Geometry: final body of the model. Coordinates: model frame, mm. A direction names the side the tool comes from. Coordinates: 2 decimals unless noted, no trailing zeros. Write each loop counter-clockwise with the first axis right and the second up, starting at its lowest first coordinate (ties: lowest second). Pieces come first, ordered by that corner, then holes. Notation, with made-up numbers: (2, 75.25) - (24, 75.25) arc R13 cw to (24, 86.25) - close; hole circle Ø6 at (-18, 33.5). An arc over 180 degrees is marked (long way). Answer as a JSON object with one key per item and string values. Group by question number.
Item 1: Section D-D on x = 16.25. Return loops of the section in (y, z).
Item 2: Set-up query: faces 1 (the flat face through (20.419, -10.108, 0.986)), 2 (the flat face through (7, 1, 0)), 3 (the flat face through (11, -14.5, 8)), 4 (the flat face through (17.875, 0, 8)), 5 (the flat face through (16, -1.5, 8)). Return all of +Z, -Z, +X, -X, +Y, -Y with unobstructed straight access to the full face (end or side cutting, diameter ignored); none if empty.
Item 3: Section A-A on z = 3.25. Return loops of the section in (x, y) (3 decimals).
Item 4: Mould query, pull axis X, two halves, no side actions, for faces 6 (the flat face through (11, 13, 8)), 7 (the flat face through (14.875, 0, 8)), 8 (the cylindrical face through (2.8, -45.89, 0.99)), 9 (the cylindrical face through (8.19, 48.22, 1.01)). Classes: pulls with the +X half, pulls with the -X half, needs draft (parallel to the pull), parting line crosses it, or undercut.
Item 5: Line query: line 1 along Y through (x, z) = (3, 1.6); line 2 along Y through (x, z) = (11, 3.5); line 3 along Z through (x, y) = (2.5, 29.5). Output: solid intervals per line, ascending. Write a range as from..to.
Item 6: Section B-B on y = 0. Return loops of the section in (x, z) (3 decimals), and give its area (3 significant figures).
Item 7: Section C-C on x = 3. Return loops of the section in (y, z), and give its area (3 significant figures).
Item 8: First-contact query: pin 1 Ø2 at (x, z) = (18.5, 13) entering from +Y; pin 2 Ø0.9 at (x, z) = (16.5, 11.5) entering from +Y; pin 3 Ø6 at (x, z) = (12, 9.5) entering from -Y. Flat tips, straight axial feed; report the tip coordinate or a pass-through.
```python
from build123d import *

# Parameters (mm, degrees)
SKETCH1_R           = 1.5
BOSS_EXTRUDE1_DEPTH = 2
FILLET1_R           = 15
FILLET2_R           = 3
FILLET3_R           = 1.5
FILLET4_R           = 5
SKETCH2_W           = 1.5
SKETCH2_H           = 3
SKETCH2_W_2         = 0.75
BOSS_EXTRUDE2_DEPTH = 13
SKETCH4_W           = 3
SKETCH4_H           = 29
CUT_EXTRUDE1_DEPTH  = 13


with BuildPart() as part:
    # Sketch1 → Boss-Extrude1 (new body)
    with BuildSketch(Plane.XY):
        Polygon((0, 52.37615434), (0, -52.37615434), (8.5, -48.47615434), (13, -20), (28, 0), (13, 20), (8.5, 48.47615434), align=None)
        with Locations((3, -47.37615434)):
            Circle(SKETCH1_R, mode=Mode.SUBTRACT)
        with Locations((22.62384566, 0)):
            Circle(SKETCH1_R, mode=Mode.SUBTRACT)
        with Locations(Location((3, 47.37615434, 0), (0, 0, 180))):
            Circle(SKETCH1_R, mode=Mode.SUBTRACT)
    extrude(amount=BOSS_EXTRUDE1_DEPTH)

    # Fillet1
    fillet1_edges = [part.edges().sort_by_distance(p)[0] for p in [
        (13, 20, 1),
        (13, -20, 1),
    ]]
    fillet(fillet1_edges, radius=FILLET1_R)

    # Fillet2
    fillet2_edges = [part.edges().sort_by_distance(p)[0] for p in [
        (8.5, 48.47615434, 1),
        (8.5, -48.47615434, 1),
    ]]
    fillet(fillet2_edges, radius=FILLET2_R)

    # Fillet3
    fillet3_edges = [part.edges().sort_by_distance(p)[0] for p in [
        (0, -52.37615434, 1),
        (0, 52.37615434, 1),
    ]]
    fillet(fillet3_edges, radius=FILLET3_R)

    # Fillet4
    fillet4_edges = [part.edges().sort_by_distance(p)[0] for p in [
        (28, 0, 1),
    ]]
    fillet(fillet4_edges, radius=FILLET4_R)

    # Sketch2 → Boss-Extrude2 (add)
    with BuildSketch(Plane.XY.offset(2)):
        Polygon((17.125, 13), (17.125, 14.5), (0, 14.5), (0, -14.5), (17.125, -14.5), (17.125, -13), (15.625, -13), (1.5, -13), (1.5, 13), (15.625, 13), align=None)
        with Locations((16.375, 0)):
            Rectangle(SKETCH2_W, SKETCH2_H)
        with Locations((17.5, 0)):
            Rectangle(SKETCH2_W_2, SKETCH2_H)
        with Locations((15.25, 0)):
            Rectangle(SKETCH2_W_2, SKETCH2_H)
    extrude(amount=BOSS_EXTRUDE2_DEPTH)

    # Sketch4 → Cut-Extrude1 (cut)
    with BuildSketch(Plane.XY.offset(15)):
        with Locations((3, 0)):
            Rectangle(SKETCH4_W, SKETCH4_H)
    extrude(amount=-CUT_EXTRUDE1_DEPTH, mode=Mode.SUBTRACT)


solid = part.part
```
Checks:
{
 "1": {"outline": "(-15.67, 0) - (15.67, 0) - (15.67, 2) - (14.5, 2) - (14.5, 15) - (13, 15) - (13, 2) - (1.5, 2) - (1.5, 15) - (-1.5, 15) - (-1.5, 2) - (-13, 2) - (-13, 15) - (-14.5, 15) - (-14.5, 2) - (-15.67, 2) - close"},
 "2": {"face 1": "+Z, -Z, +X, -Y", "face 2": "-Z, +X, -X, +Y, -Y", "face 3": "+Z, +X, -X, -Y", "face 4": "+Z, +X, +Y, -Y", "face 5": "+Z, +X"},
 "3": {"outline": "(0, -14.5) - (1.5, -14.5) - (1.5, 14.5) - (0, 14.5) - close; (4.5, -14.5) - (17.125, -14.5) - (17.125, -13) - (4.5, -13) - close; (4.5, 13) - (17.125, 13) - (17.125, 14.5) - (4.5, 14.5) - close; (14.875, -1.5) - (17.875, -1.5) - (17.875, 1.5) - (14.875, 1.5) - close"},
 "4": {"face 6": "needs draft", "face 7": "undercut", "face 8": "undercut", "face 9": "pulls with the +X half"},
 "5": {"line 1": "-51..-48.88, -45.88..45.88, 48.88..51", "line 2": "-14.5..-13, 13..14.5", "line 3": "0..2"},
 "6": {"outline": "(0, 0) - (21.124, 0) - (21.124, 2) - (17.875, 2) - (17.875, 15) - (14.875, 15) - (14.875, 2) - (1.5, 2) - (1.5, 15) - (0, 15) - close; (24.124, 0) - (26.75, 0) - (26.75, 2) - (24.124, 2) - close", "area": "106 mm^2"},
 "7": {"outline": "(-51, 0) - (-48.88, 0) - (-48.88, 2) - (-51, 2) - close; (-45.88, 0) - (45.88, 0) - (45.88, 2) - (-45.88, 2) - close; (48.88, 0) - (51, 0) - (51, 2) - (48.88, 2) - close", "area": "192 mm^2"},
 "8": {"pin 1": "y = 1.5", "pin 2": "y = 14.5", "pin 3": "y = -14.5"}
}
